from build123d import *

# Parameters (mm, degrees)
F0_W     = 13
F0_H     = 17
F1_DEPTH = 8
F2_R     = 1.7
F3_DEPTH = 6
F4_R     = 3
F5_DEPTH = 25


with BuildPart() as f1:
    # F0 (on Front) → F1 (new body)
    with BuildSketch(Plane.XZ):
        with Locations((6.5, 8.5)):
            Rectangle(F0_W, F0_H)
    extrude(amount=F1_DEPTH)

    # F2 (on face) → F3 (cut)
    with BuildSketch(Plane.XY.offset(17)):
        with Locations((3.5, -4)):
            Circle(F2_R)
        with Locations((9.5, -4)):
            Circle(F2_R)
    extrude(amount=-F3_DEPTH, mode=Mode.SUBTRACT)

    # F4 (on face) → F5 (cut)
    with BuildSketch(Plane.XZ.offset(8)):
        with Locations((6.5, 7)):
            Circle(F4_R)
    extrude(amount=-F5_DEPTH, mode=Mode.SUBTRACT)


solid = f1.part
Here's how the part is built. I have some questions about the finished solid (model axes, mm). A direction names the side the tool comes from. Give positions to 0.01 mm unless a question says otherwise; leave off trailing zeros. Loops run counter-clockwise (first coordinate to the right, second up) from the corner with the lowest first, then second, coordinate; pieces in that order, holes last. Notation, with made-up numbers: (17, 88.25) -> (38, 88.25) arc R28 ccw to (38, 117.25) -> close; hole circle Ø2 at (25, -26). An arc over 180 degrees is marked (long way). Answer as a JSON object with one key per item and string values. Group by question number.
Item 1: Imagine slicing it at A-A on x = 6.5. Write out the boundary of the cut face in (y, z), then the cut area to 3 significant figures.
Item 2: Will this pin go through, and if not, where does the flat tip stop? pin 1 (7 mm diameter, centred on x = 6.5, z = 7, fed in from -Y).
Item 3: On a 3-axis mill with a long thin cutter (end or side, diameter ignored), from which of +Z, -Z, +X, -X, +Y, -Y can I reach the whole of each face in a straight line? I mean faces 1 (the flat face through (9, -4, 11)), 2 (the flat face through (6, 0, 11)). Say none if no direction works.
Item 4: Thinking about a two-plate mould opening in Z: for faces 3 (the flat face through (3, -4, 11)), 4 (the cylindrical face through (9.27, -4.06, 5.85)), 5 (the flat face through (0, -4, 8)), 6 (the flat face through (6, -4, 0)), which applies, pulls with the +Z half, pulls with the -Z half, needs draft (parallel to the pull), parting line crosses it, or undercut?
Item 5: Imagine slicing it at B-B on y = -4. Write out the boundary of the cut face in (x, z), then the cut area to 3 significant figures.
Item 6: Imagine slicing it at C-C on z = 7. Write out the boundary of the cut face in (x, y).
Item 7: I need wall thicknesses on L1, parallel to Z at x = 6.5, y = -7.5; L2, parallel to Z at x = 4.25, y = -0.5; L3, parallel to Y at x = 3.5, z = 12.85. Which ranges of each line are inside material? Lowest first, please.
Item 8: Imagine slicing it at D-D on z = 13.5. Write out the boundary of the cut face in (x, y), then the cut area to 3 significant figures.
Answer list:
{
 "1": {"outline": "(-8, 0) -> (0, 0) -> (0, 4) -> (-8, 4) -> close; (-8, 10) -> (0, 10) -> (0, 17) -> (-8, 17) -> close", "area": "88.0 mm2"},
 "2": {"pin 1": "stops at y = -8"},
 "3": {"face 1": "+Z", "face 2": "+Z, -Z, +X, -X, +Y"},
 "4": {"face 3": "pulls with the +Z half", "face 4": "undercut", "face 5": "needs draft", "face 6": "pulls with the -Z half"},
 "5": {"outline": "(0, 0) -> (13, 0) -> (13, 17) -> (11.2, 17) -> (11.2, 11) -> (7.8, 11) -> (7.8, 17) -> (5.2, 17) -> (5.2, 11) -> (1.8, 11) -> (1.8, 17) -> (0, 17) -> close; hole circle Ø6 at (6.5, 7)", "area": "152 mm2"},
 "6": {"outline": "(0, -8) -> (3.5, -8) -> (3.5, 0) -> (0, 0) -> close; (9.5, -8) -> (13, -8) -> (13, 0) -> (9.5, 0) -> close"},
 "7": {"L1": "z = 0 to 4, 10 to 17", "L2": "z = 0 to 5.02, 8.98 to 17", "L3": "y = -8 to -5.7, -2.3 to 0"},
 "8": {"outline": "(0, -8) -> (13, -8) -> (13, 0) -> (0, 0) -> close; hole circle Ø3.4 at (3.5, -4); hole circle Ø3.4 at (9.5, -4)", "area": "85.8 mm2"}
}
